Verification items for the finished model (mm, model axes). A direction names the side the tool comes from. Give positions to 0.01 mm unless a question says otherwise; leave off trailing zeros. Order: outer loops, then holes, each group sorted by start corner. A loop starts at its lowest first (then second) coordinate and runs counter-clockwise, first axis right, second up.
from build123d import *

# Parameters (mm, degrees)
F0_R     = 2.4
F0_W     = 18
F0_H     = 4
F1_DEPTH = 5


# Not quite as in the source:
# - ends of sketch curves that miss each other by under 0.0002 mm in the source are joined


with BuildPart() as f1:
    # F0 (on Top) → F1 (new body)
    with BuildSketch(Plane.XY):
        with BuildLine():
            Line((-12.8452325787, 14), (-30, 14))
            ThreePointArc((-30, 14), (-33.5355339059, 12.5355339059), (-35, 9))
            Line((-35, 9), (-35, -9))
            ThreePointArc((-35, -9), (-33.5355339059, -12.5355339059), (-30, -14))
            Line((-30, -14), (-12.8452325787, -14))
            ThreePointArc((-12.8452325787, -14), (-19, 0), (-12.8452325787, 14))
        make_face()
        with BuildLine():
            ThreePointArc((-28.5, -2.5), (-31, 0), (-28.5, 2.5))
            Line((-28.5, 2.5), (-22.5, 2.5))
            ThreePointArc((-22.5, 2.5), (-20.7249314431, 1.7717582393), (-19.9886980778, 0))
            ThreePointArc((-19.9886980778, 0), (-20.724931484, -1.77175828), (-22.5, -2.4999744532))
            Line((-22.5, -2.4999744532), (-28.5, -2.5))
        make_face(mode=Mode.SUBTRACT)
        with BuildLine():
            Line((12.8452325787, 14), (-12.8452325787, 14))
            ThreePointArc((-12.8452325787, 14), (-19, 0), (-12.8452325787, -14))
            add(Edge.make_bspline(
                [(-9, -10), (-10.2817441929, -11.3333333333), (-11.5634883858, -12.6666666667), (-12.8452325787, -14)],
                knots=[0, 0, 0, 0, 5.5484965156, 5.5484965156, 5.5484965156, 5.5484965156], degree=3))
            Line((-9, -10), (9, -10))
            add(Edge.make_bspline(
                [(9, -10), (10.2817441929, -11.3333333333), (11.5634883858, -12.6666666667), (12.8452325787, -14)],
                knots=[0, 0, 0, 0, 5.5484965156, 5.5484965156, 5.5484965156, 5.5484965156], degree=3))
            ThreePointArc((12.8452325787, -14), (17.393381198, -7.6465868531), (19, 0))
            ThreePointArc((19, 0), (17.393381198, 7.6465868531), (12.8452325787, 14))
        make_face()
        Circle(F0_R, mode=Mode.SUBTRACT)
        with BuildLine():
            ThreePointArc((12.8452325787, 14), (0, 19), (-12.8452325787, 14))
            Line((-12.8452325787, 14), (12.8452325787, 14))
        make_face()
        with BuildLine():
            Line((30, 14), (12.8452325787, 14))
            ThreePointArc((12.8452325787, 14), (17.393381198, 7.6465868531), (19, 0))
            ThreePointArc((19, 0), (17.393381198, -7.6465868531), (12.8452325787, -14))
            Line((12.8452325787, -14), (30, -14))
            ThreePointArc((30, -14), (33.5355339059, -12.5355339059), (35, -9))
            Line((35, -9), (35, 9))
            ThreePointArc((35, 9), (33.5355339059, 12.5355339059), (30, 14))
        make_face()
        with BuildLine():
            ThreePointArc((22.5, -2.5), (20, 0), (22.5, 2.5))
            Line((22.5, 2.5), (28.5, 2.5))
            ThreePointArc((28.5, 2.5), (30.267766953, 1.767766953), (31, 0))
            ThreePointArc((31, 0), (30.267766953, -1.767766953), (28.5, -2.5))
            Line((28.5, -2.5), (22.5, -2.5))
        make_face(mode=Mode.SUBTRACT)
        with Locations((0, -12)):
            Rectangle(F0_W, F0_H)
        with BuildLine():
            add(Edge.make_bspline(
                [(-9, -10), (-10.2817441929, -11.3333333333), (-11.5634883858, -12.6666666667), (-12.8452325787, -14)],
                knots=[0, 0, 0, 0, 5.5484965156, 5.5484965156, 5.5484965156, 5.5484965156], degree=3))
            Line((-12.8452325787, -14), (-9, -14))
            Line((-9, -14), (-9, -10))
        make_face()
        with BuildLine():
            Line((9, -14), (12.8452325787, -14))
            add(Edge.make_bspline(
                [(9, -10), (10.2817441929, -11.3333333333), (11.5634883858, -12.6666666667), (12.8452325787, -14)],
                knots=[0, 0, 0, 0, 5.5484965156, 5.5484965156, 5.5484965156, 5.5484965156], degree=3))
            Line((9, -10), (9, -14))
        make_face()
    extrude(amount=F1_DEPTH)


solid = f1.part
(1) Section check A-A, the plane x = 0. Enter the section's corners in (y, z), then the cut area to 3 significant figures.
Solved:
outline: (-14, 0) - (-2.4, 0) - (-2.4, 5) - (-14, 5) - close; (2.4, 0) - (19, 0) - (19, 5) - (2.4, 5) - close
area: 141 mm2
(2) Section check C-C, the plane y = -1.5. Enter the section's corners in (x, z), then the cut area to 3 significant figures.
Solved:
outline: (-35, 0) - (-30.5, 0) - (-30.5, 5) - (-35, 5) - close; (-20.49, 0) - (-1.87, 0) - (-1.87, 5) - (-20.49, 5) - close; (1.87, 0) - (20.5, 0) - (20.5, 5) - (1.87, 5) - close; (30.5, 0) - (35, 0) - (35, 5) - (30.5, 5) - close
area: 231 mm2
(3) Set-up check for faces 1 (the flat face through (0, 3, 5)), 2 (the flat face through (22, 14, 2)), 3 (the flat face through (26, -2.5, 2)): record each of +Z, -Z, +X, -X, +Y, -Y from which the full face is reachable in a straight line by a thin tool's end or side.
Solved:
face 1: +Z, +X, -X, +Y, -Y
face 2: +Z, -Z, +X, +Y
face 3: +Z, -Z
(4) Scan lines: line 1 (Y direction, x = 25, z = 4.2); line 2 (Y direction, x = 13, z = 1.2); line 3 (Y direction, x = -29, z = 1.4). Record each from-to range of solid material in increasing order.
Solved:
line 1: y = -14 to -2.5, 2.5 to 14
line 2: y = -14 to 14
line 3: y = -14 to -2.45, 2.45 to 14
(5) Section check B-B, the plane z = 2.45. Enter the section's corners in (x, y), then the cut area to 3 significant figures.
Solved:
outline: (-35, -9) arc R5 ccw to (-30, -14) - (30, -14) arc R5 ccw to (35, -9) - (35, 9) arc R5 ccw to (30, 14) - (12.85, 14) arc R19 ccw to (-12.85, 14) - (-30, 14) arc R5 ccw to (-35, 9) - close; hole (-28.5, -2.5) - (-22.5, -2.5) arc R2.5 ccw to (-19.99, 0) arc R2.5 ccw to (-22.5, 2.5) - (-28.5, 2.5) arc R2.5 ccw to start; hole circle Ø4.8 at (0, 0); hole (22.5, -2.5) - (28.5, -2.5) arc R2.5 ccw to (28.5, 2.5) - (22.5, 2.5) arc R2.5 ccw to start
area: 1,910 mm2
(6) Section check D-D, the plane x = 15. Enter the section's corners in (y, z).
Solved:
outline: (-14, 0) - (14, 0) - (14, 5) - (-14, 5) - close
(7) Release check for a two-part mould opening along Y. For faces 4 (the flat face through (35, 0, 2)), 5 (the cylindrical face through (-20.745, 1.791, 2.465)), 6 (the cylindrical face through (-33, 13, 2)) record: pulls with the +Y half, pulls with the -Y half, needs draft (parallel to the pull), parting line crosses it, or undercut.
Solved:
face 4: needs draft
face 5: undercut
face 6: pulls with the +Y half
(8) Go/stop test with flat-tipped pins: pin 1 (3 mm diameter, centred on x = -20, y = 2.5, fed in from -Z); pin 2 (2.5 mm diameter, centred on x = -19, z = 1.5, fed in from +Y). Record where each tip stops, or that it passes through.
Solved:
pin 1: stops at z = 0
pin 2: stops at y = 14
